Work out the finished part from the listing and answer in its coordinate system (mm). A direction names the side the tool comes from. Give positions to 0.01 mm unless a question says otherwise; leave off trailing zeros. Order: outer loops, then holes, each group sorted by start corner. A loop starts at its lowest first (then second) coordinate and runs counter-clockwise, first axis right, second up. Notation, with made-up numbers: (34, 13) - (49, 13) arc R21 ccw to (49, 48) - close; hole circle Ø5 at (33.25, -6.75). An arc over 180 degrees is marked (long way). Put each result on its own line as item: value.
```python
from build123d import *

# Parameters (mm, degrees)
F1_DEPTH = 26
F3_DEPTH = 200
F4_SIZE2 = 2
F4_SIZE  = 2
F5_D     = 5
F5_DEPTH = 300
F5_START = 15.25
F5_TIP   = 1.5021515476
F8_D     = 7
F8_DEPTH = 300
F8_TIP   = 2.1030121666


with BuildPart() as f1:
    # F0 (on Front) → F1 (new body)
    with BuildSketch(Plane.XZ):
        Polygon((-71.2336192391, 8.5), (-71.2336192391, 0), (92.2663807609, 0), (92.2663807609, 8.5), (77.0163807609, 8.5), (77.0163807609, 29), (72.0163807609, 29), (72.0163807609, 8.5), (13.0163807609, 8.5), (13.0163807609, 29), (8.0163807609, 29), (8.0163807609, 8.5), (-50.9836192391, 8.5), (-50.9836192391, 29), (-55.9836192391, 29), (-55.9836192391, 8.5), align=None)
    extrude(amount=F1_DEPTH)

    # F2 (on face) → F3 (cut)
    with BuildSketch(Plane.YZ.offset(92.2663807609)):
        with BuildLine():
            ThreePointArc((-13, 1.9879535556), (-19.5755600396, 1.4880932085), (-26, 0))
            Line((-26, 0), (-13, 0))
            Line((-13, 0), (-13, 1.9879535556))
        make_face()
        with BuildLine():
            ThreePointArc((0, 0), (-6.4244399604, 1.4880932085), (-13, 1.9879535556))
            Line((-13, 1.9879535556), (-13, 0))
            Line((-13, 0), (0, 0))
        make_face()
    extrude(amount=-F3_DEPTH, mode=Mode.SUBTRACT)

    # F4
    f4_edges = [f1.edges().sort_by_distance(p)[0] for p in [
        (74.516381, 0, 29),
        (74.516381, -26, 29),
        (10.516381, -26, 29),
        (10.516381, 0, 29),
        (-53.483619, -26, 29),
        (-53.483619, 0, 29),
    ]]
    chamfer(f4_edges, length=F4_SIZE, length2=F4_SIZE2)

    # F5
    # its depths count from where the whole tool has entered the part; down to there all is cleared
    with Locations(Plane.YZ.offset(92.2663807609).offset(-F5_START)):
        with Locations((-20, 18.7), (-6, 18.7)):
            Hole(F5_D / 2, depth=F5_DEPTH)
            with Locations((0, 0, -(F5_DEPTH + F5_TIP / 2))):  # 118° drill point
                Cone(0, F5_D / 2, F5_TIP, mode=Mode.SUBTRACT)

    # F8
    with Locations(Plane.XY.offset(8.5)):
        with Locations((-21.4836192391, -13), (42.5163807609, -13)):
            Hole(F8_D / 2, depth=F8_DEPTH)
            with Locations((0, 0, -(F8_DEPTH + F8_TIP / 2))):  # 118° drill point
                Cone(0, F8_D / 2, F8_TIP, mode=Mode.SUBTRACT)


solid = f1.part
```
(1) Section B-B, the plane y = -20 is taken. Write down the section's boundary in (x, z), then the cut area to 3 significant figures.
Geometry check:
outline: (-71.23, 1.42) - (92.27, 1.42) - (92.27, 8.5) - (77.02, 8.5) - (77.02, 16.2) - (72.02, 16.2) - (72.02, 8.5) - (13.02, 8.5) - (13.02, 16.2) - (8.02, 16.2) - (8.02, 8.5) - (-50.98, 8.5) - (-50.98, 16.2) - (-55.98, 16.2) - (-55.98, 8.5) - (-71.23, 8.5) - close; (-55.98, 21.2) - (-50.98, 21.2) - (-50.98, 29) - (-55.98, 29) - close; (8.02, 21.2) - (13.02, 21.2) - (13.02, 29) - (8.02, 29) - close; (72.02, 21.2) - (77.02, 21.2) - (77.02, 29) - (72.02, 29) - close
area: 1,390 mm²
(2) Determine the mould class of faces 6 (the face through (9, 0, 8)), 7 (the face through (9, -26, 8)), 8 (the face through (75, -13, 29)), 9 (the face through (10.48, -7.15, 16.48)) for opening direction Y: pulls with the +Y half, pulls with the -Y half, needs draft (parallel to the pull), parting line crosses it, or undercut.
Geometry check:
face 6: pulls with the +Y half
face 7: pulls with the -Y half
face 8: needs draft
face 9: undercut
(3) Given pin 1 (4 mm diameter, centred on y = -3.5, z = 13, fed in from -X); pin 2 (7.5 mm diameter, centred on x = 86.5, y = -16, fed in from +Z); pin 3 (10 mm diameter, centred on y = -11, z = 21.5, fed in from +X), each flat-ended and moving along its own axis, determine where each tip first touches the part or whether it passes through.
Geometry check:
pin 1: stops at x = -55.98
pin 2: stops at z = 8.5
pin 3: stops at x = 77.02
(4) A tool of negligible diameter and unlimited length cuts with its end or side. For faces 1 (the face through (77.016, -13, 19)), 2 (the face through (-55.984, -13, 19)), 3 (the face through (43, -7, 8.5)), 4 (the face through (-53.5, -18, 17.2)), 5 (the face through (-53, -13, 29)), from which of +Z, -Z, +X, -X, +Y, -Y can it reach the whole face along a straight path? Write none if from no direction.
Geometry check:
face 1: +Z, +X, +Y, -Y
face 2: +Z, -X, +Y, -Y
face 3: +Z, +Y, -Y
face 4: +X, -X
face 5: +Z, +X, -X, +Y, -Y
(5) Section A-A, the plane z = 22.75 is taken. Write down the section's boundary in (x, y).
Geometry check:
outline: (-55.98, -26) - (-50.98, -26) - (-50.98, 0) - (-55.98, 0) - close; (8.02, -26) - (13.02, -26) - (13.02, 0) - (8.02, 0) - close; (72.02, -26) - (77.02, -26) - (77.02, 0) - (72.02, 0) - close
(6) Section C-C, the plane z = 3.5 is taken. Write down the section's boundary in (x, y).
Geometry check:
outline: (-71.23, -26) - (92.27, -26) - (92.27, 0) - (-71.23, 0) - close; hole circle Ø7 at (-21.48, -13); hole circle Ø7 at (42.52, -13)
(7) Straight lines are drawn through the part: line 1 (X direction, y = -6.25, z = 21.75); line 2 (X direction, y = -14.5, z = 6.75); line 3 (Z direction, x = -52.45, y = -20). For each, find the intervals that lie inside material, in ascending order.
Geometry check:
line 1: x = -55.98 to -50.98, 8.02 to 13.02, 72.02 to 77.02
line 2: x = -71.23 to -24.65, -18.32 to 39.35, 45.68 to 92.27
line 3: z = 1.42 to 16.2, 21.2 to 29
(8) Section D-D, the plane x = 30.5 is taken. Write down the section's boundary in (y, z).
Geometry check:
outline: (-26, 0) arc R43.5 cw to (0, 0) - (0, 8.5) - (-26, 8.5) - close
